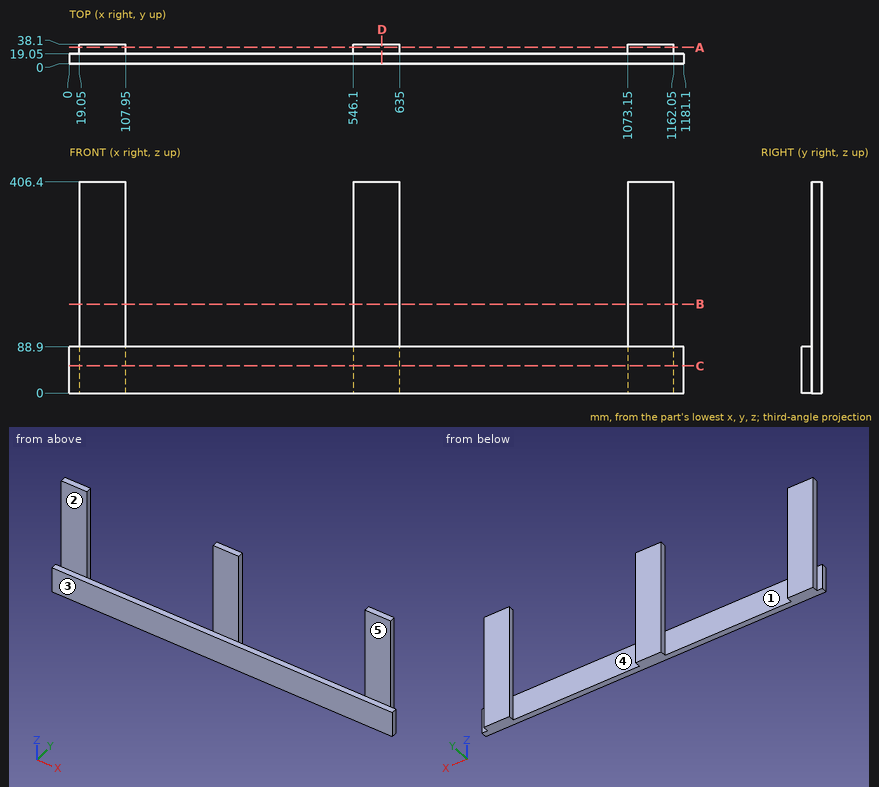
Source: three-view drawing plus pictorial views. Frame: mm from the lowest corner of the part. A direction names the side the tool comes from. Round coordinates to 2 decimals unless told otherwise and drop trailing zeros. Write each loop counter-clockwise with the first axis right and the second up, starting at its lowest first coordinate (ties: lowest second). Pieces come first, ordered by that corner, then holes. Notation, with made-up numbers: M 63,59 L 86,59 A26 ccw 86,73 Z; hole C 84.25,58.5 d9. An arc over 180 degrees is marked long. Use CSV: the item, a comma, the result in double quotes. Start each with the question number.
Q1. Access query for the marked faces 3, 4 and 5. Directions: +Z, -Z, +X, -X, +Y, -Y. A direction counts if a zero-diameter tool reaches every point of the face in a straight line with its end or side. Return the directions, or none.
Q2. Cut plane B-B on z = 171. Output: boundary loops of the cut face in (x, y).
Q3. Cut plane D-D on x = 600.5. Output: boundary loops of the cut face in (y, z).
Q4. Cut plane C-C on z = 52.5. Output: boundary loops of the cut face in (x, y), plus the area to 3 significant figures.
Q5. Line query: line 1 (X direction, y = 36.5, z = 232.5); line 2 (Y direction, x = 595, z = 160.5); line 3 (Z direction, x = 147, y = 15.5). Output: solid intervals per line, ascending. Write a range as from..to.
Q6. Pull-direction query (X, two-part tool) for the marked faces 1 and 2; classes: +X half, -X half, draft (parallel to the pull), parting line (faces both ways), or undercut.
Q7. First-contact query: P1, Ø15, axis at y = 32.5, z = 211, coming from the -X side; P2, Ø9.5, axis at x = 818, y = 8.5, coming from the +Z side; P3, Ø3, axis at y = 31.5, z = 149, coming from the +X side. Flat tips, straight axial feed; report the tip coordinate or a pass-through.
Q8. Cut plane A-A on y = 31.5. Output: boundary loops of the cut face in (x, z).
Results found:
1,face 3,"+Z, -Z, +X, -X, -Y"
1,face 4,"+Z, -Z, +Y"
1,face 5,"+Z, +X, -X, -Y"
2,outline,"M 19.05,19.05 L 107.95,19.05 L 107.95,38.1 L 19.05,38.1 Z; M 546.1,19.05 L 635,19.05 L 635,38.1 L 546.1,38.1 Z; M 1073.15,19.05 L 1162.05,19.05 L 1162.05,38.1 L 1073.15,38.1 Z"
3,outline,"M 0,0 L 38.1,0 L 38.1,406.4 L 19.05,406.4 L 19.05,88.9 L 0,88.9 Z"
4,outline,"M 0,0 L 1181.1,0 L 1181.1,19.05 L 1162.05,19.05 L 1162.05,38.1 L 1073.15,38.1 L 1073.15,19.05 L 635,19.05 L 635,38.1 L 546.1,38.1 L 546.1,19.05 L 107.95,19.05 L 107.95,38.1 L 19.05,38.1 L 19.05,19.05 L 0,19.05 Z"
4,area,"27,600 mm^2"
5,line 1,"19.05..107.95, 546.1..635, 1073.15..1162.05"
5,line 2,"19.05..38.1"
5,line 3,"0..88.9"
6,face 1,"undercut"
6,face 2,"draft"
7,P1,"x = 19.05"
7,P2,"z = 88.9"
7,P3,"x = 1162.05"
8,outline,"M 19.05,0 L 107.95,0 L 107.95,406.4 L 19.05,406.4 Z; M 546.1,0 L 635,0 L 635,406.4 L 546.1,406.4 Z; M 1073.15,0 L 1162.05,0 L 1162.05,406.4 L 1073.15,406.4 Z"
